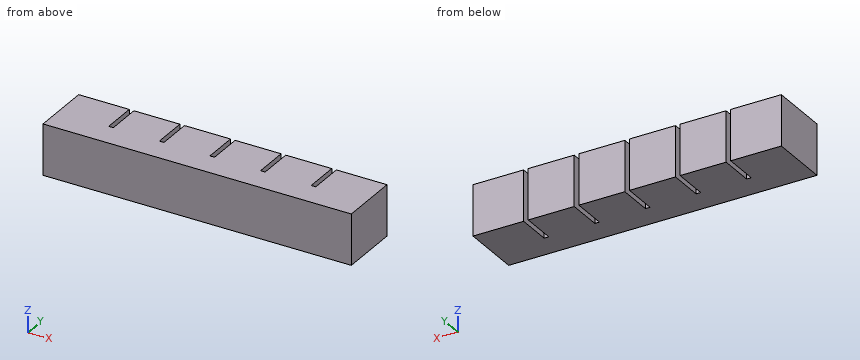
```python
from build123d import *

# Parameters (mm, degrees)
SKETCH1_W           = 20
SKETCH1_H           = 20
BOSS_EXTRUDE1_DEPTH = 22
SKETCH2_W           = 8
SKETCH2_H           = 10
CUT_EXTRUDE1_DEPTH  = 14
SKETCH3_W           = 22
SKETCH3_H           = 5
BOSS_EXTRUDE2_DEPTH = 2
LPATTERN1_COUNT     = 6
LPATTERN1_PITCH     = 22
SKETCH4_W           = 22
SKETCH4_H           = 15
BOSS_EXTRUDE3_DEPTH = 2
SKETCH5_W           = 22
SKETCH5_H           = 20
BOSS_EXTRUDE4_DEPTH = 2
SKETCH6_W           = 118
SKETCH6_H           = 2
CUT_EXTRUDE2_DEPTH  = 2
SKETCH7_W           = 134
SKETCH7_H           = 22
BOSS_EXTRUDE5_DEPTH = 6


with BuildPart() as part:
    # Sketch1 → Boss-Extrude1 (new body)
    with BuildSketch(Plane.XY):
        with Locations((10, 10)):
            Rectangle(SKETCH1_W, SKETCH1_H)
    extrude(amount=BOSS_EXTRUDE1_DEPTH)

    # Sketch2 → Cut-Extrude1 (cut)
    with BuildSketch(Plane.XZ):
        with Locations((10, 11)):
            Rectangle(SKETCH2_W, SKETCH2_H)
    extrude(amount=-CUT_EXTRUDE1_DEPTH, mode=Mode.SUBTRACT)

    # Sketch3 → Boss-Extrude2 (add)
    with BuildSketch(Plane(origin=(20, 0, 0), x_dir=(0, 0, -1), z_dir=(1, 0, 0))):
        with Locations((-11, 2.5)):
            Rectangle(SKETCH3_W, SKETCH3_H)
    extrude(amount=BOSS_EXTRUDE2_DEPTH)


with BuildPart() as lpattern1_1:
    # LPattern1: pattern copy
    add(part.part.moved(Location(Vector(1, 0, 0) * (1 * LPATTERN1_PITCH))))


with BuildPart() as lpattern1_2:
    # LPattern1: pattern copy
    add(part.part.moved(Location(Vector(1, 0, 0) * (2 * LPATTERN1_PITCH))))


with BuildPart() as lpattern1_3:
    # LPattern1: pattern copy
    add(part.part.moved(Location(Vector(1, 0, 0) * (3 * LPATTERN1_PITCH))))


with BuildPart() as lpattern1_4:
    # LPattern1: pattern copy
    add(part.part.moved(Location(Vector(1, 0, 0) * (4 * LPATTERN1_PITCH))))


with BuildPart() as lpattern1_5:
    # LPattern1: pattern copy
    add(part.part.moved(Location(Vector(1, 0, 0) * (5 * LPATTERN1_PITCH))))


with BuildPart() as lpattern1_1_1:
    add(lpattern1_1.part)

    # Combine1: union LPattern1_2, LPattern1_3, LPattern1_4, LPattern1_5, part
    add(lpattern1_2.part)
    add(lpattern1_3.part)
    add(lpattern1_4.part)
    add(lpattern1_5.part)
    add(part.part)

    # Sketch4 → Boss-Extrude3 (add)
    with BuildSketch(Plane(origin=(130, 0, 0), x_dir=(0, 0, -1), z_dir=(1, 0, 0))):
        with Locations((-11, 12.5)):
            Rectangle(SKETCH4_W, SKETCH4_H)
    extrude(amount=BOSS_EXTRUDE3_DEPTH)

    # Sketch5 → Boss-Extrude4 (add)
    with BuildSketch(Plane.ZY):
        with Locations((11, 10)):
            Rectangle(SKETCH5_W, SKETCH5_H)
    extrude(amount=BOSS_EXTRUDE4_DEPTH)

    # Sketch6 → Cut-Extrude2 (cut)
    with BuildSketch(Plane(origin=(0, 0, 0), x_dir=(-1, 0, 0), z_dir=(0, -1, 0))):
        with Locations((-65, -11)):
            Rectangle(SKETCH6_W, SKETCH6_H)
    extrude(amount=-CUT_EXTRUDE2_DEPTH, mode=Mode.SUBTRACT)

    # Sketch7 → Boss-Extrude5 (add)
    with BuildSketch(Plane(origin=(0, 0, 0), x_dir=(-1, 0, 0), z_dir=(0, -1, 0))):
        with Locations((-65, -11)):
            Rectangle(SKETCH7_W, SKETCH7_H)
    extrude(amount=BOSS_EXTRUDE5_DEPTH)


solid = lpattern1_1_1.part
```
Input: part model. Units: mm. Frame: model coordinates. Round coordinates to 2 decimals unless told otherwise and drop trailing zeros. Loops run counter-clockwise (first coordinate to the right, second up) from the corner with the lowest first, then second, coordinate; pieces in that order, holes last.
1) Section query C-C on x = 7.5. Return the cut outline in (y, z).
Ans:
outline: (-6, 0) - (20, 0) - (20, 22) - (-6, 22) - close; hole (0, 6) - (14, 6) - (14, 16) - (0, 16) - close
2) Material intervals for line 1 (X direction, y = 16.5, z = 1.75); line 2 (Z direction, x = 18, y = 1.25); line 3 (Y direction, x = 122.5, z = 14.75), sorted ascending.
Ans:
line 1: x = -2 to 20, 22 to 42, 44 to 64, 66 to 86, 88 to 108, 110 to 132
line 2: z = 0 to 10, 12 to 22
line 3: y = -6 to 0, 14 to 20
3) Section query D-D on y = 9.5. Count the separate pieces of the cut face and the enclosed holes in it, plus the area to 3 significant figures.
Ans:
separate pieces: 6
enclosed holes: 6
area: 2,250 mm2
4) Pin query (flat end, axial travel): pin 1 (1.6 mm diameter, centred on x = 43.5, z = 11.5, fed in from +Y); pin 2 (1.6 mm diameter, centred on x = 87, z = 14, fed in from +Y). Return the tip coordinate at first contact, or that it passes through.
Ans:
pin 1: stops at y = 20
pin 2: stops at y = 5
5) Section query A-A on y = 17.5. Return the cut outline in (x, z).
Ans:
outline: (-2, 0) - (20, 0) - (20, 22) - (-2, 22) - close; (22, 0) - (42, 0) - (42, 22) - (22, 22) - close; (44, 0) - (64, 0) - (64, 22) - (44, 22) - close; (66, 0) - (86, 0) - (86, 22) - (66, 22) - close; (88, 0) - (108, 0) - (108, 22) - (88, 22) - close; (110, 0) - (132, 0) - (132, 22) - (110, 22) - close
6) Section query B-B on y = 3.75. Return the cut outline in (x, z).
Ans:
outline: (-2, 0) - (132, 0) - (132, 22) - (-2, 22) - close; hole (6, 6) - (14, 6) - (14, 16) - (6, 16) - close; hole (28, 6) - (36, 6) - (36, 16) - (28, 16) - close; hole (50, 6) - (58, 6) - (58, 16) - (50, 16) - close; hole (72, 6) - (80, 6) - (80, 16) - (72, 16) - close; hole (94, 6) - (102, 6) - (102, 16) - (94, 16) - close; hole (116, 6) - (124, 6) - (124, 16) - (116, 16) - close
